The model under review builds one solid part; all positions refer to its coordinate system, in mm. A direction names the side the tool comes from. Coordinates: 2 decimals unless noted, no trailing zeros. Order: outer loops, then holes, each group sorted by start corner. A loop starts at its lowest first (then second) coordinate and runs counter-clockwise, first axis right, second up. Notation, with made-up numbers: (58.25, 53) -> (100.25, 53) arc R27 ccw to (100.25, 77) -> close; hole circle Ø5 at (88, 85). An arc over 180 degrees is marked (long way). Use one line per item in the form item = value. Start each with the question number.
(1) Insertion check: pin 1 Ø1 at (y, z) = (37.5, 7.5) entering from +X; pin 2 Ø0.6 at (x, z) = (49, 13) entering from +Y; pin 3 Ø1.5 at (x, z) = (40.5, 16.5) entering from +Y. Each pin has a flat end and moves straight along its axis. Give the tip position at first contact, or say it passes through.
(2) Take a section at C-C (x = 42). State the section outline as (y, z) points.
(3) For faces 1 (the conical face through (47.48, 7.685, 0.242)), 2 (the conical face through (48.13, 29.03, 19.85)), 3 (the flat face through (19.652, 26, 10)), list the 3-axis set-ups (+Z, -Z, +X, -X, +Y, -Y) from which the entire face can be reached by the end or side of a thin tool; tool diameter is ignored.
(4) Take a section at D-D (y = 38.5). State the section outline as (x, z) points, then the cut area to 3 significant figures.
(5) Take a section at B-B (z = 17). State the section outline as (x, y) points.
(6) Mouldability with a two-part tool opening along X and no side actions: class faces 4 (the conical face through (48.13, 29.03, 0.15)), 5 (the cylindrical face through (17.437, 5.296, 10.134)), 6 (the conical face through (49.68, 5.46, 19.85)) as +X half, -X half, draft (parallel to the pull), parting line (faces both ways), or undercut.
(7) Wall thickness on line 1 along X through (y, z) = (20, 11.5); line 2 along X through (y, z) = (30.5, 13.5); line 3 along Y through (x, z) = (43, 18.5): over which ranges is each line inside the solid? List them lowest first.
(8) Take a section at A-A (y = 25.5). State the section outline as (x, z) points.
```python
from build123d import *

# Parameters (mm, degrees)
PAD_DEPTH    = 20
FILLET_R     = 1
CHAMFER_SIZE = 0.4


with BuildPart() as part:
    # Sketch → Pad (new body)
    with BuildSketch(Plane.XY):
        Polygon((17.151947, 44.9952), (17.151947, 4.9952), (50.151947, 4.9952), (50.151947, 29.4952), (47.651947, 29.4952), (47.651947, 7.4952), (19.651947, 7.4952), (19.651947, 44.9952), align=None)
    extrude(amount=PAD_DEPTH)

    # Fillet
    fillet_edges = [part.edges().sort_by_distance(p)[0] for p in [
        (50.151947, 4.9952, 10),
        (17.151947, 4.9952, 10),
        (19.651947, 7.4952, 10),
        (17.151947, 44.9952, 10),
        (19.651947, 44.9952, 10),
        (47.651947, 7.4952, 10),
        (47.651947, 29.4952, 10),
        (50.151947, 29.4952, 10),
    ]]
    fillet(fillet_edges, radius=FILLET_R)

    # Chamfer
    chamfer_edges = [part.edges().sort_by_distance(p)[0] for p in [
        (17.151947, 24.9952, 20),
        (17.44484, 44.702307, 20),
        (17.44484, 5.288093, 20),
        (18.401947, 44.9952, 20),
        (33.651947, 4.9952, 20),
        (19.359054, 44.702307, 20),
        (49.859054, 5.288093, 20),
        (19.651947, 26.2452, 20),
        (50.151947, 17.2452, 20),
        (19.94484, 7.788093, 20),
        (49.859054, 29.202307, 20),
        (33.651947, 7.4952, 20),
        (48.901947, 29.4952, 20),
        (47.359054, 7.788093, 20),
        (47.94484, 29.202307, 20),
        (47.651947, 18.4952, 20),
        (17.151947, 24.9952, 0),
        (17.44484, 44.702307, 0),
        (17.44484, 5.288093, 0),
        (18.401947, 44.9952, 0),
        (33.651947, 4.9952, 0),
        (19.359054, 44.702307, 0),
        (49.859054, 5.288093, 0),
        (19.651947, 26.2452, 0),
        (50.151947, 17.2452, 0),
        (19.94484, 7.788093, 0),
        (49.859054, 29.202307, 0),
        (33.651947, 7.4952, 0),
        (48.901947, 29.4952, 0),
        (47.359054, 7.788093, 0),
        (47.94484, 29.202307, 0),
        (47.651947, 18.4952, 0),
    ]]
    chamfer(chamfer_edges, length=CHAMFER_SIZE)


solid = part.part
```
Findings:
q1.pin_1 = 19.65
q1.pin_2 = 29.5
q1.pin_3 = 7.5
q2.outline = (5, 0.4) -> (5.4, 0) -> (7.1, 0) -> (7.5, 0.4) -> (7.5, 19.6) -> (7.1, 20) -> (5.4, 20) -> (5, 19.6) -> close
q3.face_1 = -Z, +Y
q3.face_2 = +Z, +Y
q3.face_3 = +Z, -Z, +Y
q4.outline = (17.15, 0.4) -> (17.55, 0) -> (19.25, 0) -> (19.65, 0.4) -> (19.65, 19.6) -> (19.25, 20) -> (17.55, 20) -> (17.15, 19.6) -> close
q4.area = 49.7 mm²
q5.outline = (17.15, 6) arc R1 ccw to (18.15, 5) -> (49.15, 5) arc R1 ccw to (50.15, 6) -> (50.15, 28.5) arc R1 ccw to (49.15, 29.5) -> (48.65, 29.5) arc R1 ccw to (47.65, 28.5) -> (47.65, 8.5) arc R1 cw to (46.65, 7.5) -> (20.65, 7.5) arc R1 cw to (19.65, 8.5) -> (19.65, 44) arc R1 ccw to (18.65, 45) -> (18.15, 45) arc R1 ccw to (17.15, 44) -> close
q6.face_4 = undercut
q6.face_5 = -X half
q6.face_6 = +X half
q7.line_1 = 17.15 to 19.65, 47.65 to 50.15
q7.line_2 = 17.15 to 19.65
q7.line_3 = 5 to 7.5
q8.outline = (17.15, 0.4) -> (17.55, 0) -> (19.25, 0) -> (19.65, 0.4) -> (19.65, 19.6) -> (19.25, 20) -> (17.55, 20) -> (17.15, 19.6) -> close; (47.65, 0.4) -> (48.05, 0) -> (49.75, 0) -> (50.15, 0.4) -> (50.15, 19.6) -> (49.75, 20) -> (48.05, 20) -> (47.65, 19.6) -> close
